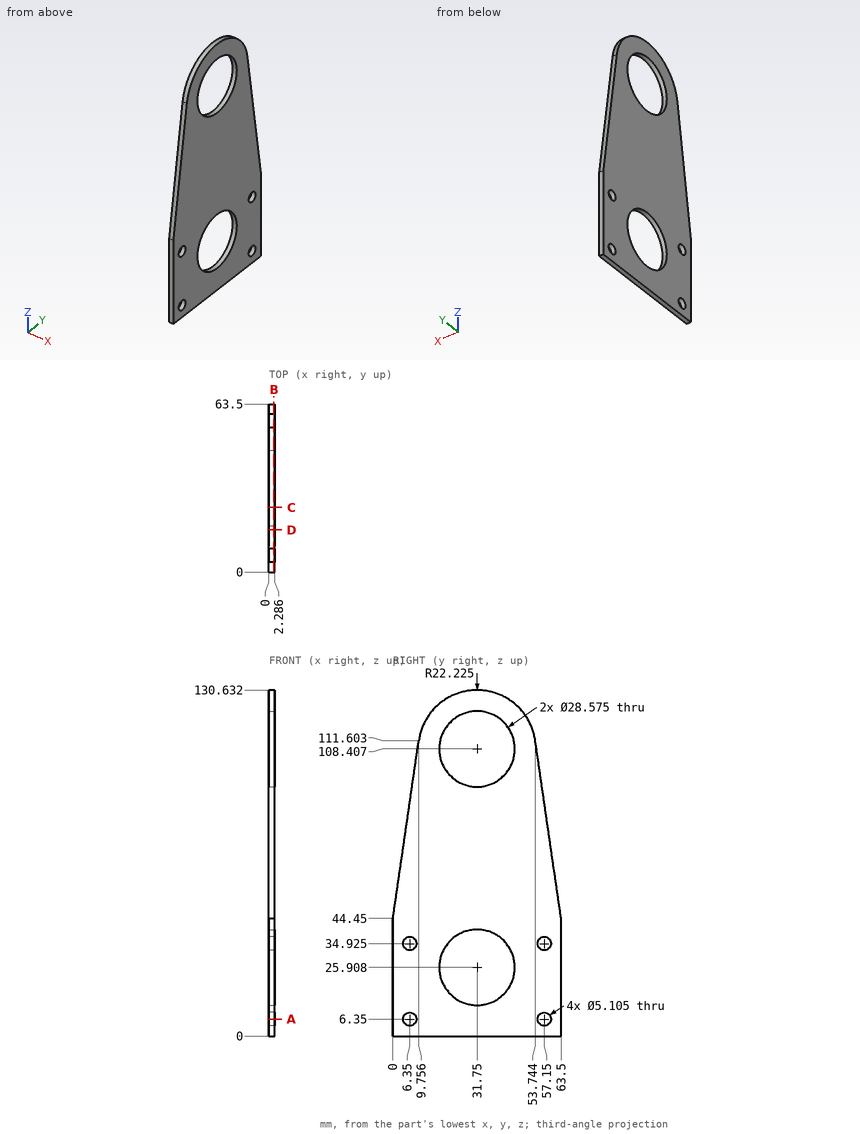
Check sheet for the drawn part. Datum: minimum x, y, z corner. Units: mm. Coordinates: 2 decimals unless noted, no trailing zeros. Order: outer loops, then holes, each group sorted by start corner. A loop starts at its lowest first (then second) coordinate and runs counter-clockwise, first axis right, second up. Notation, with made-up numbers: M 20,-20.5 L 40,-20.5 A36 cw 40,15.5 Z; hole C 19,73 d2. An arc over 180 degrees is marked long. One line per question, with ' | ' between items. Start each with the question number.
Item 1: Sectioned sample at C-C on y = 24.5. Record the cut outline in (x, z) (1 decimal), and give its area (3 significant figures).
Item 2: Sectioned sample at D-D on y = 16. Record the cut outline in (x, z) (1 decimal).
Item 3: Sectioned sample at B-B on x = 1.85. Count the separate pieces of the cut face and the enclosed holes in it, and give its area (3 significant figures).
Item 4: Gauge pin test, flat end, axial feed: P1, Ø1, axis at x = 0.5, z = 77, coming from the -Y side. Record the tip position at first contact, or that the pin passes through.
Item 5: Sectioned sample at A-A on z = 6.35. Record the cut outline in (x, y) (1 decimal).
Item 6: Material ranges on line 1 (Y direction, x = 1.5, z = 6.35); line 2 (Z direction, x = 0.75, y = 31.75) (1 decimal); line 3 (Z direction, x = 1.6, y = 29), recorded low to high.
Answer below:
1) outline: M 0,0 L 2.3,0 L 2.3,13.6 L 0,13.6 Z; M 0,38.2 L 2.3,38.2 L 2.3,96.1 L 0,96.1 Z; M 0,120.7 L 2.3,120.7 L 2.3,129.4 L 0,129.4 Z | area: 183 mm^2
2) outline: M 0,0 L 2.3,0 L 2.3,124.1 L 0,124.1 Z
3) separate pieces: 1 | enclosed holes: 6 | area: 5,700 mm^2
4) P1: stops at y = 4.66
5) outline: M 0,0 L 2.3,0 L 2.3,3.8 L 0,3.8 Z; M 0,8.9 L 2.3,8.9 L 2.3,54.6 L 0,54.6 Z; M 0,59.7 L 2.3,59.7 L 2.3,63.5 L 0,63.5 Z
6) line 1: y = 0 to 3.8, 8.9 to 54.6, 59.7 to 63.5 | line 2: z = 0 to 11.6, 40.2 to 94.1, 122.7 to 130.6 | line 3: z = 0 to 11.89, 39.93 to 94.39, 122.43 to 130.46
